```python
from build123d import *

# Parameters (mm, degrees)
BOSS_EXTRUDE1_DEPTH = 63.3
FILLET1_R           = 1
FILLET2_R           = 1
FILLET3_R           = 1
FILLET4_R           = 1
FILLET20_R          = 1
FILLET21_R          = 1
FILLET22_R          = 1
FILLET23_R          = 1


with BuildPart() as part:
    # Sketch1 → Boss-Extrude1 (new body)
    with BuildSketch(Plane(origin=(0, 0, 0), x_dir=(1, 0, 0), z_dir=(0, 1, 0))):
        with BuildLine():
            Line((-0.8, -0.8), (-0.8, -2.102974084))
            ThreePointArc((-0.8, -2.102974084), (0, -2.25), (0.8, -2.102974084))
            Line((0.8, -2.102974084), (0.8, -0.8))
            Line((0.8, -0.8), (2.102974084, -0.8))
            ThreePointArc((2.102974084, -0.8), (2.25, 0), (2.102974084, 0.8))
            Line((2.102974084, 0.8), (0.8, 0.8))
            Line((0.8, 0.8), (0.8, 2.102974084))
            ThreePointArc((0.8, 2.102974084), (0, 2.25), (-0.8, 2.102974084))
            Line((-0.8, 2.102974084), (-0.8, 0.8))
            Line((-0.8, 0.8), (-2.102974084, 0.8))
            ThreePointArc((-2.102974084, 0.8), (-2.25, 0), (-2.102974084, -0.8))
            Line((-2.102974084, -0.8), (-0.8, -0.8))
        make_face()
    extrude(amount=BOSS_EXTRUDE1_DEPTH)

    # Fillet1
    fillet1_edges = [part.edges().sort_by_distance(p)[0] for p in [
        (-2.25, 0, 0),
    ]]
    fillet(fillet1_edges, radius=FILLET1_R)

    # Fillet2
    fillet2_edges = [part.edges().sort_by_distance(p)[0] for p in [
        (0, 0, 2.25),
    ]]
    fillet(fillet2_edges, radius=FILLET2_R)

    # Fillet3
    fillet3_edges = [part.edges().sort_by_distance(p)[0] for p in [
        (2.25, 0, 0),
    ]]
    fillet(fillet3_edges, radius=FILLET3_R)

    # Fillet4
    fillet4_edges = [part.edges().sort_by_distance(p)[0] for p in [
        (0, 0, -2.25),
    ]]
    fillet(fillet4_edges, radius=FILLET4_R)

    # Fillet20
    fillet20_edges = [part.edges().sort_by_distance(p)[0] for p in [
        (2.25, 63.3, 0),
    ]]
    fillet(fillet20_edges, radius=FILLET20_R)

    # Fillet21
    fillet21_edges = [part.edges().sort_by_distance(p)[0] for p in [
        (0, 63.3, 2.25),
    ]]
    fillet(fillet21_edges, radius=FILLET21_R)

    # Fillet22
    fillet22_edges = [part.edges().sort_by_distance(p)[0] for p in [
        (-2.25, 63.3, 0),
    ]]
    fillet(fillet22_edges, radius=FILLET22_R)

    # Fillet23
    fillet23_edges = [part.edges().sort_by_distance(p)[0] for p in [
        (0, 63.3, -2.25),
    ]]
    fillet(fillet23_edges, radius=FILLET23_R)


solid = part.part
```
Build history of the part. All positions in model axes, mm. A direction names the side the tool comes from. Round coordinates to 2 decimals unless told otherwise and drop trailing zeros. Write each loop counter-clockwise with the first axis right and the second up, starting at its lowest first coordinate (ties: lowest second). Pieces come first, ordered by that corner, then holes. Notation, with made-up numbers: (24, -24.5) - (55, -24.5) arc R7 cw to (55, -17.5) - close; hole circle Ø10 at (79.25, 26). An arc over 180 degrees is marked (long way). Write each question's results on one line, items separated by ' | '. Start each with the question number.
Item 1: Saw through at A-A (y = 58). Write the cut outline in (x, z), and give its area (3 significant figures).
Item 2: Wall check: L1, parallel to Z at x = -1.85, y = 15; L2, parallel to Z at x = -0.1, y = 37.5. Give the ranges that are in metal, low to high. Write a range as [from, to].
Item 3: Which spindle directions (+Z, -Z, +X, -X, +Y, -Y) get a long thin tool onto all of the face, cutting with end or side? Do faces 1 (the face through (1, 31, -0.8)), 2 (the face through (-1, 31, -0.8)), 3 (the face through (0.8, 31, 1)). Say none if no direction does.
Item 4: Drop flat-ended pins along their axis: P1, Ø1.4, axis at y = 34, z = -1, coming from the +X side; P2, Ø1, axis at x = -1.5, y = 16, coming from the -Z side; P3, Ø1, axis at y = 24, z = -1.5, coming from the -X side. Give the stop position or say it passes through.
Results are:
1) outline: (-2.1, -0.8) - (-0.8, -0.8) - (-0.8, -2.1) arc R2.25 ccw to (0.8, -2.1) - (0.8, -0.8) - (2.1, -0.8) arc R2.25 ccw to (2.1, 0.8) - (0.8, 0.8) - (0.8, 2.1) arc R2.25 ccw to (-0.8, 2.1) - (-0.8, 0.8) - (-2.1, 0.8) arc R2.25 ccw to start | area: 11.5 mm²
2) L1: z = [-0.8, 0.8] | L2: z = [-2.25, 2.25]
3) face 1: -Z, +X, +Y, -Y | face 2: -Z, -X, +Y, -Y | face 3: +Z, +X, +Y, -Y
4) P1: stops at x = 2.23 | P2: stops at z = -0.8 | P3: stops at x = -0.8
